from build123d import *

# Parameters (mm, degrees)
SKETCH1_W           = 40
SKETCH1_H           = 8
SKETCH1_W_2         = 9
SKETCH1_R           = 2.05
BOSS_EXTRUDE1_DEPTH = 2
SKETCH1_3_W         = 40
SKETCH1_3_H         = 8
BOSS_EXTRUDE2_DEPTH = 9
FILLET1_R           = 4
FILLET2_R           = 1
FILLET4_R           = 1.5
FILLET5_R           = 1


with BuildPart() as part:
    # Sketch1 → Boss-Extrude1 (new body)
    # profile 1 of 3: a face of its own
    with BuildSketch(Plane(origin=(0, 0, 0), x_dir=(1, 0, 0), z_dir=(0, 1, 0))):
        with Locations((29, -4)):
            Rectangle(SKETCH1_W, SKETCH1_H)
    # profile 2 of 3: a face of its own
    with BuildSketch(Plane(origin=(0, 0, 0), x_dir=(1, 0, 0), z_dir=(0, 1, 0))):
        with Locations((4.5, -4)):
            Rectangle(SKETCH1_W_2, SKETCH1_H)
        with Locations(Location((4.5, -4, 0), (0, 0, 270))):
            Circle(SKETCH1_R, mode=Mode.SUBTRACT)
    # profile 3 of 3: a face of its own
    with BuildSketch(Plane(origin=(0, 0, 0), x_dir=(1, 0, 0), z_dir=(0, 1, 0))):
        with Locations((53.5, -4)):
            Rectangle(SKETCH1_W_2, SKETCH1_H)
        with Locations(Location((53.5, -4, 0), (0, 0, 270))):
            Circle(SKETCH1_R, mode=Mode.SUBTRACT)
    extrude(amount=BOSS_EXTRUDE1_DEPTH)

    # Sketch1<3> → Boss-Extrude2 (add)
    with BuildSketch(Plane(origin=(0, 0, 0), x_dir=(1, 0, 0), z_dir=(0, 1, 0))):
        with Locations((29, -4)):
            Rectangle(SKETCH1_3_W, SKETCH1_3_H)
    extrude(amount=BOSS_EXTRUDE2_DEPTH)

    # Fillet1
    fillet1_edges = [part.edges().sort_by_distance(p)[0] for p in [
        (29, 9, 0),
        (29, 9, 8),
    ]]
    fillet(fillet1_edges, radius=FILLET1_R - 0.0001)  # a hair under: the kernel refuses the full size

    # Fillet2
    fillet2_edges = [part.edges().sort_by_distance(p)[0] for p in [
        (0, 1, 8),
        (0, 1, 0),
        (58, 1, 0),
        (58, 1, 8),
    ]]
    fillet(fillet2_edges, radius=FILLET2_R)

    # Fillet4
    fillet4_edges = [part.edges().sort_by_distance(p)[0] for p in [
        (9, 2, 4),
        (49, 2, 4),
    ]]
    fillet(fillet4_edges, radius=FILLET4_R)

    # Fillet5
    fillet5_edges = [part.edges().sort_by_distance(p)[0] for p in [
        (9, 4.25005, 0),
        (49, 4.25005, 0),
        (49, 4.25005, 8),
        (49, 7.828456414, 6.828456414),
        (49, 7.828456414, 1.171543586),
        (9, 4.25005, 8),
        (9, 7.828456414, 6.828456414),
        (9, 7.828456414, 1.171543586),
        (4.25, 2, 0),
        (58, 2, 4),
        (57.707106781, 2, 7.707106781),
        (57.707106781, 2, 0.292893219),
        (4.25, 2, 8),
        (0, 2, 4),
        (0.292893219, 2, 7.707106781),
        (0.292893219, 2, 0.292893219),
        (53.75, 2, 0),
        (53.75, 2, 8),
        (49.439339828, 2.439339828, 0),
        (49.439339828, 2.439339828, 8),
        (8.560660172, 2.439339828, 0),
        (8.560660172, 2.439339828, 8),
    ]]
    fillet(fillet5_edges, radius=FILLET5_R)


solid = part.part
CAD build for the part. Positions are in the model's coordinates, mm. A direction names the side the tool comes from. Give positions to 0.01 mm unless a question says otherwise; leave off trailing zeros. Write each loop counter-clockwise with the first axis right and the second up, starting at its lowest first coordinate (ties: lowest second). Pieces come first, ordered by that corner, then holes. Notation, with made-up numbers: (53, 64) -> (109, 64) arc R32 ccw to (109, 100) -> close; hole circle Ø2 at (-28, -39.75). An arc over 180 degrees is marked (long way). Return JSON: item names as keys, results as strings.
Item 1: Band-saw the part on B-B (y = 0.5). List the corners of the cut face in (x, z).
Answer below:
{"outline": "(0, 1) arc R1 ccw to (1, 0) -> (57, 0) arc R1 ccw to (58, 1) -> (58, 7) arc R1 ccw to (57, 8) -> (1, 8) arc R1 ccw to (0, 7) -> close; hole circle Ø4.1 at (4.5, 4); hole circle Ø4.1 at (53.5, 4)"}
Item 2: Two-plate mould, pull along X, no slides. Class faces 5 (the cylindrical face through (3.253, 0.986, 2.373)), 6 (the cylindrical face through (0.301, 1.715, 3.958)), 7 (the flat face through (54.43, 2, 1.96)): +X half, -X half, draft (parallel to the pull), parting line (faces both ways), or undercut.
Answer below:
{"face 5": "undercut", "face 6": "-X half", "face 7": "draft"}
Item 3: Band-saw the part on A-A (x = 53.5). List the corners of the cut face in (y, z).
Answer below:
{"outline": "(0, 0) -> (1, 0) arc R1 ccw to (2, 1) -> (2, 1.95) -> (0, 1.95) -> close; (0, 6.05) -> (2, 6.05) -> (2, 7) arc R1 ccw to (1, 8) -> (0, 8) -> close"}
Item 4: Band-saw the part on D-D (z = 3.25). Give the number of separate pieces and of enclosed holes in the cut face, then the cut area to 3 significant figures.
Answer below:
{"separate pieces": "3", "enclosed holes": "0", "area": "378 mm2"}
Item 5: Drill centre lines: probe 1 along X at (y, z) = (0.5, 4); probe 2 along Y at (x, z) = (31, 4.25); probe 3 along X at (y, z) = (4.25, 7). Where is each one in solid material? Low to high.
Answer below:
{"probe 1": "x = 0 to 2.45, 6.55 to 51.45, 55.55 to 58", "probe 2": "y = 0 to 8.99", "probe 3": "x = 9 to 49"}
Item 6: Tool access for faces 1 (the cylindrical face through (4.204, 1.715, 7.699)), 2 (the cylindrical face through (48.715, 4.24, 7.699)), 3 (the cylindrical face through (48.715, 4.261, 0.301)), 4 (the cylindrical face through (9.285, 4.261, 0.301)): list every direction of +Z, -Z, +X, -X, +Y, -Y with a clear straight run to the whole face (end or side of a thin tool).
Answer below:
{"face 1": "+Z, -X, +Y", "face 2": "+Z, +X, +Y", "face 3": "-Z, +X, +Y", "face 4": "-Z, -X, +Y"}
Item 7: Drop flat-ended pins along their axis: pin 1 (3 mm diameter, centred on x = 52.5, z = 3.5, fed in from +Y); pin 2 (3.5 mm diameter, centred on x = 53.5, z = 4, fed in from -Y); pin 3 (1.5 mm diameter, centred on x = 13, y = 7.5, fed in from -Z); pin 4 (2 mm diameter, centred on y = 4.5, z = 4.5, fed in from +X). Give the stop position or say it passes through.
Answer below:
{"pin 1": "stops at y = 2", "pin 2": "passes through", "pin 3": "stops at z = 0.4", "pin 4": "stops at x = 49"}
